Here's the drawing with two shaded views (mm, measured from the low corner). I have some questions. Coordinates: 2 decimals unless noted, no trailing zeros. Loops run counter-clockwise (first coordinate to the right, second up) from the corner with the lowest first, then second, coordinate; pieces in that order, holes last. Notation, with made-up numbers: (19.5, 2) -> (51.5, 2) arc R20 ccw to (51.5, 35) -> close; hole circle Ø11 at (38, 29). An arc over 180 degrees is marked (long way). Use CSV: the item, a comma, the result in double quotes. Start each with the question number.
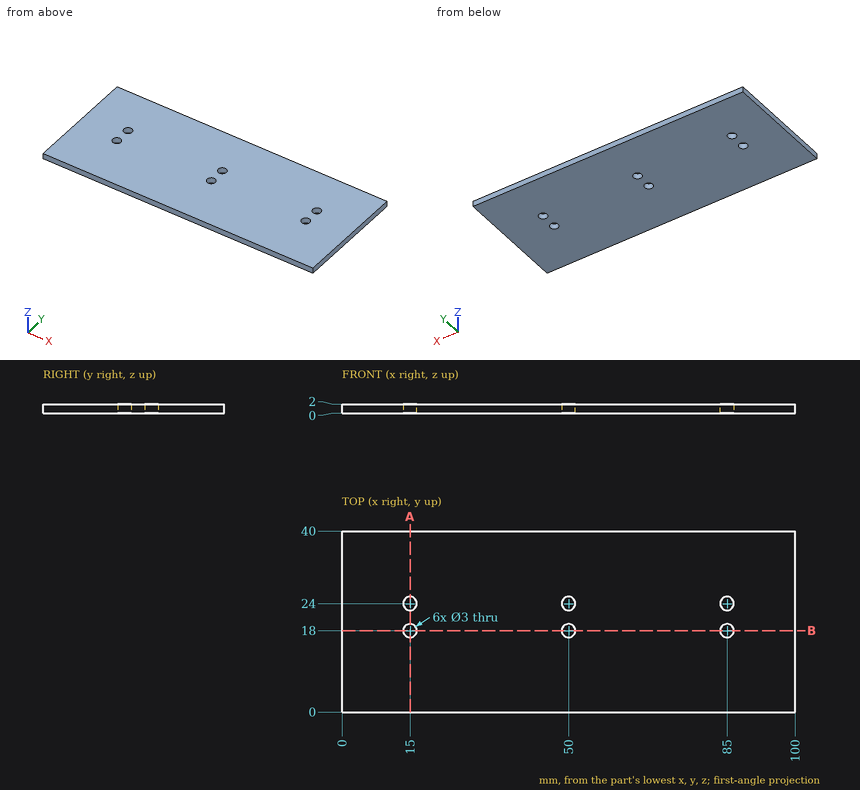
1) I want a section at A-A, the plane x = 15. Please give me the cut outline in (y, z).
2) Please list where these lines run through material, in increasing order: L1, parallel to Y at x = 15, z = 1.05; L2, parallel to Y at x = 84, z = 0.45; L3, parallel to X at y = 23.5, z = 1.55. Write a range as [from, to].
3) I want a section at B-B, the plane y = 18. Please give me the cut outline in (x, z), plus the area to 3 significant figures.
Return value:
1,outline,"(0, 0) -> (16.5, 0) -> (16.5, 2) -> (0, 2) -> close; (19.5, 0) -> (22.5, 0) -> (22.5, 2) -> (19.5, 2) -> close; (25.5, 0) -> (40, 0) -> (40, 2) -> (25.5, 2) -> close"
2,L1,"y = [0, 16.5], [19.5, 22.5], [25.5, 40]"
2,L2,"y = [0, 16.88], [19.12, 22.88], [25.12, 40]"
2,L3,"x = [0, 13.59], [16.41, 48.59], [51.41, 83.59], [86.41, 100]"
3,outline,"(0, 0) -> (13.5, 0) -> (13.5, 2) -> (0, 2) -> close; (16.5, 0) -> (48.5, 0) -> (48.5, 2) -> (16.5, 2) -> close; (51.5, 0) -> (83.5, 0) -> (83.5, 2) -> (51.5, 2) -> close; (86.5, 0) -> (100, 0) -> (100, 2) -> (86.5, 2) -> close"
3,area,"182 mm²"
